Autodesk Inventor part; units mm, degrees
ref_plane "YZ Plane" through (0, 0, 0) normal (1, 0, 0) x (0, 1, 0)
ref_plane "XZ Plane" through (0, 0, 0) normal (0, 1, 0) x (-1, 0, 0)
ref_plane "XY Plane" through (0, 0, 0) normal (0, 0, 1) x (1, 0, 0)
sketch "Sketch1" plane through (0, 0, 0) normal (0, 0, 1) x (1, 0, 0)
  circle A0 centre (0, 0) radius 4
  dimension "Diameter" = 8
extrude "Extrusion1" add sketch "Sketch1" along normal blind 90
sketch "Sketch2" plane through (0, 0, 90) normal (0, 0, 1) x (1, 0, 0)
  circle A0 centre (0, 0) radius 4
  circle A1 centre (0, 0) radius 6.5
  dimension "Head_Diameter" = 13
extrude "Extrusion2" add sketch "Sketch2" along normal blind 8 contours A0 | A1
sketch "Sketch3" plane through (0, 0, 98) normal (0, 0, 1) x (1, 0, 0)
  circle A0 centre (0, 0) radius 6.5
  circle A1 centre (0, 0) radius 3.4641 construction
  line L0 (0, 3.4641) -> (3, 1.7321)
  line L1 (3, -1.7321) -> (3, 1.7321)
  line L2 (0, 3.4641) -> (-3, 1.7321)
  line L3 (-3, -1.7321) -> (-3, 1.7321)
  line L4 (-3, -1.7321) -> (0, -3.4641)
  line L5 (3, -1.7321) -> (0, -3.4641)
  dimension "Hex_Width" = 6
extrude "Extrusion3" cut sketch "Sketch3" against normal blind 4 contours L0 L1 L5 L4 L3 L2
thread "Thread1"
chamfer "Chamfer1" distance 0.8 angle 45 2 edges at (-6.5, 0, 98) (-4, 0, 0)
equation "\"d9\" = ThreadLength"
equation "\"d12\" = Chamfer"
equation "\"ThreadLength\" = 28"
properties part number "SCREW,SOCKET HD,P,12.9,M8X1.25X90MM"
Geometry: final body of the model. Coordinates: model frame, mm. A direction names the side the tool comes from. Give positions to 0.01 mm unless a question says otherwise; leave off trailing zeros. Loops run counter-clockwise (first coordinate to the right, second up) from the corner with the lowest first, then second, coordinate; pieces in that order, holes last. Notation, with made-up numbers: M 50.5,-12 L 100.5,-12 A22 cw 100.5,1 Z; hole C 73.25,60.5 d8. An arc over 180 degrees is marked long. Put each result on its own line as item: value. Start each with the question number.
1) Pull-direction query (Y, two-part tool) for faces 4 (the cylindrical face through (-0.867, 3.905, 44.776)), 5 (the flat face through (-3, 0, 96)), 6 (the flat face through (0, 0, 0)), 7 (the flat face through (1.5, -2.6, 96)); classes: pulls with the +Y half, pulls with the -Y half, needs draft (parallel to the pull), parting line crosses it, or undercut.
2) Ray query, line 1 along Z through (x, y) = (-1.75, 1); line 2 along Z through (x, y) = (0.25, -4.75); line 3 along X through (y, z) = (-0.25, 63). Return the intervals inside material, ascending.
3) Cut plane B-B (z = 11). Output: boundary loops of the cut face in (x, y).
4) Cut plane A-A (y = 0). Output: boundary loops of the cut face in (x, z), then the cut area to 3 significant figures.
5) Contact query for flat-ended pins moving along their axis: pin 1 (5 mm diameter, centred on y = -3, z = 46, fed in from -X); pin 2 (1.7 mm diameter, centred on y = -1, z = 96.5, fed in from +X); pin 3 (2 mm diameter, centred on y = -3, z = 59, fed in from -X). Output: stop coordinate, or through.
6) Access query for faces 1 (the cylindrical face through (-5.158, 3.955, 93.55)), 2 (the flat face through (3, 3, 90)), 3 (the flat face through (-1.5, -2.6, 96)). Directions: +Z, -Z, +X, -X, +Y, -Y. A direction counts if a zero-diameter tool reaches every point of the face in a straight line with its end or side. Return the directions, or none.
Verdict:
1. face 4: parting line crosses it
1. face 5: undercut
1. face 6: needs draft
1. face 7: undercut
2. line 1: 0 to 94
2. line 2: 90 to 98
2. line 3: -3.99 to 3.99
3. outline: C 0,0 d8
4. outline: M -6.5,90 L -4,90 L -4,0.8 L -3.2,0 L 3.2,0 L 4,0.8 L 4,90 L 6.5,90 L 6.5,97.2 L 5.7,98 L 3,98 L 3,94 L -3,94 L -3,98 L -5.7,98 L -6.5,97.2 Z
4. area: 799 mm2
5. pin 1: x = -3.97
5. pin 2: x = 6.5
5. pin 3: x = -3.46
6. face 1: +Z, -Z
6. face 2: -Z
6. face 3: +Z
